Could you check a few things on this drawing? It's one solid part, dimensions in mm from its lowest x, y, z. A direction names the side the tool comes from. Coordinates: 2 decimals unless noted, no trailing zeros. Order: outer loops, then holes, each group sorted by start corner. A loop starts at its lowest first (then second) coordinate and runs counter-clockwise, first axis right, second up.
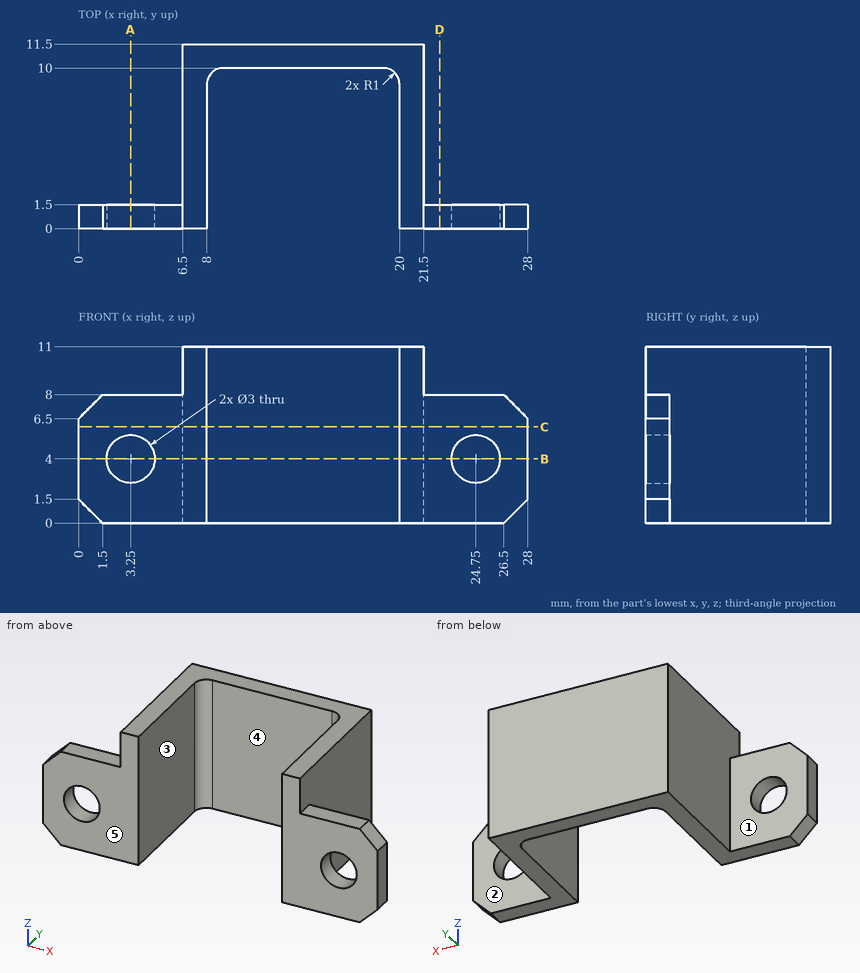
Q1. If we section it at B-B on z = 4: Write out the boundary of the cut face in (x, y).
Q2. We'd pull the mould along X, two halves only. Please class the marked faces 4 and 5: pulls with the +X half, pulls with the -X half, needs draft (parallel to the pull), parting line crosses it, or undercut.
Q3. For the marked faces 1, 2 and 3, which set-ups out of +Z, -Z, +X, -X, +Y, -Y let a thin tool reach every point of the face, with its end or its side?
Q4. If we section it at D-D on x = 22.5: Write out the boundary of the cut face in (y, z).
Q5. I need wall thicknesses on L1, parallel to X at y = 3, z = 8.5; L2, parallel to Z at x = 24.75, y = 0.95; L3, parallel to Y at x = 12, z = 7.75. Which ranges of each line are inside material? Lowest first, please.
Q6. If we section it at C-C on z = 6: Write out the boundary of the cut face in (x, y).
Q7. Will these pins go through, and if not, where does the flat tip stop? pin 1 (3 mm diameter, centred on y = 4, z = 3, fed in from +X); pin 2 (5 mm diameter, centred on x = 14.5, z = 3.5, fed in from -Y); pin 3 (1.2 mm diameter, centred on x = 23.5, y = 1, fed in from +Z); pin 4 (2.5 mm diameter, centred on x = 3.25, z = 4, fed in from -Y).
Q8. If we section it at A-A on x = 3.25: Write out the boundary of the cut face in (y, z).
Reply:
1. outline: (0, 0) - (1.75, 0) - (1.75, 1.5) - (0, 1.5) - close; (4.75, 0) - (8, 0) - (8, 9) arc R1 cw to (9, 10) - (19, 10) arc R1 cw to (20, 9) - (20, 0) - (23.25, 0) - (23.25, 1.5) - (21.5, 1.5) - (21.5, 11.5) - (6.5, 11.5) - (6.5, 1.5) - (4.75, 1.5) - close; (26.25, 0) - (28, 0) - (28, 1.5) - (26.25, 1.5) - close
2. face 4: undercut
2. face 5: needs draft
3. face 1: +Z, -Z, -X, +Y
3. face 2: +Z, -Z, +X, +Y
3. face 3: +Z, -Z, -Y
4. outline: (0, 0) - (1.5, 0) - (1.5, 8) - (0, 8) - close
5. L1: x = 6.5 to 8, 20 to 21.5
5. L2: z = 0 to 2.5, 5.5 to 8
5. L3: y = 10 to 11.5
6. outline: (0, 0) - (8, 0) - (8, 9) arc R1 cw to (9, 10) - (19, 10) arc R1 cw to (20, 9) - (20, 0) - (28, 0) - (28, 1.5) - (21.5, 1.5) - (21.5, 11.5) - (6.5, 11.5) - (6.5, 1.5) - (0, 1.5) - close
7. pin 1: stops at x = 21.5
7. pin 2: stops at y = 10
7. pin 3: stops at z = 8
7. pin 4: passes through
8. outline: (0, 0) - (1.5, 0) - (1.5, 2.5) - (0, 2.5) - close; (0, 5.5) - (1.5, 5.5) - (1.5, 8) - (0, 8) - close
